Part model, mm, in its own coordinate system. Round coordinates to 2 decimals unless told otherwise and drop trailing zeros. Write each loop counter-clockwise with the first axis right and the second up, starting at its lowest first coordinate (ties: lowest second). Pieces come first, ordered by that corner, then holes. Notation, with made-up numbers: M -37,-33 L 15,-33 A16 cw 15,-29 Z; hole C -18.5,-11.5 d5. An arc over 180 degrees is marked long. Answer as a JSON object with one key per item and string values. Group by question number.
1. Drop flat-ended pins along their axis: pin 1 (1.5 mm diameter, centred on y = -5, z = -2, fed in from -X); pin 2 (3 mm diameter, centred on y = -3.5, z = -2, fed in from -X). Give the stop position or say it passes through.
2. Band-saw the part on A-A, the plane y = -2. Count the separate pieces of the cut face and the enclosed holes in it, plus the area to 3 significant figures.
3. Two-plate mould, pull along Z, no slides. Class faces 1 (the face through (0, -3, -3.5)), 2 (the face through (-3, -7, 0)), 3 (the face through (-10, -4, 0)): +Z half, -Z half, draft (parallel to the pull), parting line (faces both ways), or undercut.
4. Band-saw the part on B-B, the plane x = 24. Write the cut outline in (y, z), plus the area to 3 significant figures.
5. Drill centre lines: line 1 (Z direction, x = -23.5, y = -2.75); line 2 (Z direction, x = -16, y = -4); line 3 (X direction, y = -4.25, z = -3). Where is each one in solid material? Low to high. Write a range as from..to.
6. Band-saw the part on D-D, the plane x = -8. Write the cut outline in (y, z), plus the area to 3 significant figures.
from build123d import *

# Parameters (mm, degrees)
F1_DEPTH = 7
F4_DEPTH = 7.001


with BuildPart() as f1:
    # F0 (on Front) → F1 (new body)
    with BuildSketch(Plane.XZ):
        with BuildLine():
            Line((-31.5, -3.5), (31.5, -3.5))
            ThreePointArc((31.5, -3.5), (33.974874, -2.474874), (35, 0))
            ThreePointArc((35, 0), (33.974874, 2.474874), (31.5, 3.5))
            Line((31.5, 3.5), (-31.5, 3.5))
            ThreePointArc((-31.5, 3.5), (-33.974874, 2.474874), (-35, 0))
            ThreePointArc((-35, 0), (-33.974874, -2.474874), (-31.5, -3.5))
        make_face()
    extrude(amount=F1_DEPTH)

    # F3 (on face) → F4 (cut, through all)
    with BuildSketch(Plane.XZ.offset(7)):
        with BuildLine():
            ThreePointArc((28.556413, 0), (31.056413, -2.5), (33.556413, 0))
            Line((33.556413, 0), (28.556413, 0))
        make_face()
        with BuildLine():
            Line((28.556413, 0), (33.556413, 0))
            ThreePointArc((33.556413, 0), (31.056413, 2.5), (28.556413, 0))
        make_face()
        with BuildLine():
            ThreePointArc((-34, 0), (-31.5, -2.5), (-29, 0))
            Line((-29, 0), (-34, 0))
        make_face()
        with BuildLine():
            Line((-34, 0), (-29, 0))
            ThreePointArc((-29, 0), (-31.5, 2.5), (-34, 0))
        make_face()
        with BuildLine():
            ThreePointArc((-26, 0), (-23.5, -2.5), (-21, 0))
            Line((-21, 0), (-26, 0))
        make_face()
        with BuildLine():
            Line((-26, 0), (-21, 0))
            ThreePointArc((-21, 0), (-23.5, 2.5), (-26, 0))
        make_face()
        with BuildLine():
            ThreePointArc((-18, 0), (-15.5, -2.5), (-13, 0))
            Line((-13, 0), (-18, 0))
        make_face()
        with BuildLine():
            Line((-18, 0), (-13, 0))
            ThreePointArc((-13, 0), (-15.5, 2.5), (-18, 0))
        make_face()
        with BuildLine():
            ThreePointArc((-10, 0), (-7.5, -2.5), (-5, 0))
            Line((-5, 0), (-10, 0))
        make_face()
        with BuildLine():
            Line((-10, 0), (-5, 0))
            ThreePointArc((-5, 0), (-7.5, 2.5), (-10, 0))
        make_face()
        with BuildLine():
            ThreePointArc((-2.5, 0), (0, -2.5), (2.5, 0))
            Line((2.5, 0), (-2.5, 0))
        make_face()
        with BuildLine():
            Line((-2.5, 0), (2.5, 0))
            ThreePointArc((2.5, 0), (0, 2.5), (-2.5, 0))
        make_face()
        with BuildLine():
            ThreePointArc((5.5, 0), (8, -2.5), (10.5, 0))
            Line((10.5, 0), (5.5, 0))
        make_face()
        with BuildLine():
            Line((5.5, 0), (10.5, 0))
            ThreePointArc((10.5, 0), (8, 2.5), (5.5, 0))
        make_face()
        with BuildLine():
            ThreePointArc((13.5, 0), (16, -2.5), (18.5, 0))
            Line((18.5, 0), (13.5, 0))
        make_face()
        with BuildLine():
            Line((13.5, 0), (18.5, 0))
            ThreePointArc((18.5, 0), (16, 2.5), (13.5, 0))
        make_face()
        with BuildLine():
            ThreePointArc((21.5, 0), (24, -2.5), (26.5, 0))
            Line((26.5, 0), (21.5, 0))
        make_face()
        with BuildLine():
            Line((21.5, 0), (26.5, 0))
            ThreePointArc((26.5, 0), (24, 2.5), (21.5, 0))
        make_face()
    extrude(amount=-F4_DEPTH, mode=Mode.SUBTRACT)


solid = f1.part
Worked answers:
{
 "1": {"pin 1": "stops at x = -34.77", "pin 2": "stops at x = -34.96"},
 "2": {"separate pieces": "1", "enclosed holes": "9", "area": "303 mm^2"},
 "3": {"face 1": "-Z half", "face 2": "draft", "face 3": "undercut"},
 "4": {"outline": "M -7,-3.5 L 0,-3.5 L 0,-2.5 L -7,-2.5 Z; M -7,2.5 L 0,2.5 L 0,3.5 L -7,3.5 Z", "area": "14.0 mm^2"},
 "5": {"line 1": "z = -3.5..-2.5, 2.5..3.5", "line 2": "z = -3.5..-2.45, 2.45..3.5", "line 3": "x = -33.3..33.3"},
 "6": {"outline": "M -7,-3.5 L 0,-3.5 L 0,-2.45 L -7,-2.45 Z; M -7,2.45 L 0,2.45 L 0,3.5 L -7,3.5 Z", "area": "14.7 mm^2"}
}
